Source: CAD feature listing. Evaluate the final solid. Frame: model axes, mm. Face numbers are marked on the shaded views. A direction names the side the tool comes from. Round coordinates to 2 decimals unless told otherwise and drop trailing zeros. Order: outer loops, then holes, each group sorted by start corner. A loop starts at its lowest first (then second) coordinate and runs counter-clockwise, first axis right, second up. Notation, with made-up numbers: M 80,22 L 125,22 A20 cw 125,51 Z; hole C 65.5,15 d2. An arc over 180 degrees is marked long. Answer as CSV lines item,"result". Start each with the question number.
Item 1: Section query C-C on y = 15. Return the cut outline in (x, z), plus the area to 3 significant figures.
Item 2: Set-up query: the marked faces 1 and 2. Return all of +Z, -Z, +X, -X, +Y, -Y with unobstructed straight access to the full face (end or side cutting, diameter ignored); none if empty.
Item 3: Pull-direction query (Z, two-part tool) for the marked faces 3, 4, 5 and 6; classes: +Z half, -Z half, draft (parallel to the pull), parting line (faces both ways), or undercut.
Item 4: Section query A-A on z = 43. Return the cut outline in (x, y), plus the area to 3 significant figures.
Item 5: Line query: line 1 (Y direction, x = -12.5, z = 23); line 2 (Y direction, x = -20, z = 2). Output: solid intervals per line, ascending. Write a range as [from, to].
Item 6: Section query B-B on x = 0. Return the cut outline in (y, z), plus the area to 3 significant figures.
Item 7: First-contact query: P1, Ø2.5, axis at y = 11.5, z = 2.5, coming from the +X side; P2, Ø1.1, axis at x = 27, z = 16, coming from the +Y side; P3, Ø3, axis at x = 20, y = 15, coming from the +Z side; P4, Ø4, axis at x = 9.9, z = 52.9, coming from the +Y side. Flat tips, straight axial feed; report the tip coordinate or a pass-through.
Item 8: Section query D-D on y = 23.25. Return the cut outline in (x, z).
from build123d import *

# Parameters (mm, degrees)
SKETCH016_W         = 54
SKETCH016_H         = 20
SKETCH016_R         = 2.35
PAD010_DEPTH        = 5
SKETCH019_R         = 11.1
SKETCH019_R_2       = 1.65
PAD009_DEPTH        = 10
SKETCH017_R         = 32.6
POCKET006_DEPTH     = 15.001
SKETCH076_R         = 32.6
SKETCH076_R_2       = 28.75
PAD049_DEPTH        = 4
SKETCH090_R         = 1.092
PAD055_DEPTH        = 26.5
HOLE009_D           = 3.4
HOLE009_CSINK_D     = 6.7
HOLE009_CSINK_ANGLE = 90


with BuildPart() as part:
    # Sketch016 → Pad010 (new body)
    with BuildSketch(Plane.XY):
        with Locations((0, 10)):
            Rectangle(SKETCH016_W, SKETCH016_H)
        with Locations((-20, 15)):
            Circle(SKETCH016_R, mode=Mode.SUBTRACT)
        with Locations((20, 15)):
            Circle(SKETCH016_R, mode=Mode.SUBTRACT)
    extrude(amount=PAD010_DEPTH)

    # Sketch019 → Pad009 (join)
    with BuildSketch(Plane.XZ):
        with BuildLine():
            Line((-27, 5), (-34.41436, 34.287835))
            ThreePointArc((34.41436, 34.287835), (0, 78.5), (-34.41436, 34.287835))
            Line((34.41436, 34.287835), (27, 5))
            Line((-27, 5), (27, 5))
        make_face()
        with Locations((0, 43)):
            Circle(SKETCH019_R, mode=Mode.SUBTRACT)
        with Locations((9.899495, 52.899495)):
            Circle(SKETCH019_R_2, mode=Mode.SUBTRACT)
        with Locations((-9.899495, 52.899495)):
            Circle(SKETCH019_R_2, mode=Mode.SUBTRACT)
        with Locations((9.899495, 33.100505)):
            Circle(SKETCH019_R_2, mode=Mode.SUBTRACT)
        with Locations((-9.899495, 33.100505)):
            Circle(SKETCH019_R_2, mode=Mode.SUBTRACT)
    extrude(amount=-PAD009_DEPTH)

    # Sketch017 → Pocket006 (cut, through all)
    with BuildSketch(Plane.XZ.offset(-5)):
        with Locations((0, 43)):
            Circle(SKETCH017_R)
    extrude(amount=-POCKET006_DEPTH, mode=Mode.SUBTRACT)

    # Sketch076 → Pad049 (join)
    with BuildSketch(Plane.XZ.offset(-4)):
        with Locations((0, 43)):
            Circle(SKETCH076_R)
        with Locations((0, 43)):
            Circle(SKETCH076_R_2, mode=Mode.SUBTRACT)
    extrude(amount=-PAD049_DEPTH)

    # Sketch090 → Pad055 (join)
    with BuildSketch(Plane.XZ):
        Polygon((28.284271, 24.615224), (23.334524, 19.665476), (23.334524, 12.594408), (32.526912, 3.40202), (41.012193, 11.887302), align=None)
        with Locations((32.526912, 10.473088)):
            Circle(SKETCH090_R, mode=Mode.SUBTRACT)
        with Locations((26.870058, 16.129942)):
            Circle(SKETCH090_R, mode=Mode.SUBTRACT)
    extrude(amount=-PAD055_DEPTH)

    # Hole009 (through all)
    with Locations(Plane(origin=(0, 5, 0), x_dir=(1, 0, 0), z_dir=(0, 1, 0))):
        with Locations((-9.899495, -52.899495), (9.899495, -52.899495), (9.899495, -33.100505), (-9.899495, -33.100505)):
            CounterSinkHole(HOLE009_D / 2, HOLE009_CSINK_D / 2, counter_sink_angle=HOLE009_CSINK_ANGLE)


solid = part.part
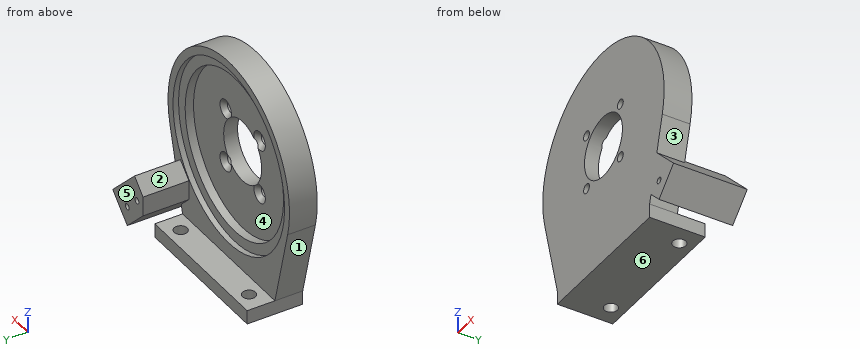
Results:
1,outline,"M -27,0 L -22.35,0 L -22.35,5 L -27,5 Z; M -17.65,0 L 17.65,0 L 17.65,5 L -17.65,5 Z; M 22.35,0 L 27,0 L 27,5 L 22.35,5 Z; M 23.33,12.59 L 32.53,3.4 L 41.01,11.89 L 28.28,24.62 L 23.33,19.67 Z; hole C 26.87,16.13 d2.18; hole C 32.53,10.47 d2.18"
1,area,"419 mm^2"
2,face 1,"-Z, -X, +Y, -Y"
2,face 2,"+Z, -X, +Y"
3,face 3,"undercut"
3,face 4,"undercut"
3,face 5,"draft"
3,face 6,"-Z half"
4,outline,"M -35.5,0 L -11.1,0 L -11.1,5 L -28.75,5 L -28.75,8 L -32.6,8 L -32.6,10 L -35.5,10 Z; M 11.1,0 L 35.5,0 L 35.5,10 L 32.6,10 L 32.6,8 L 28.75,8 L 28.75,5 L 11.1,5 Z"
4,area,"296 mm^2"
5,line 1,"[0, 5]"
5,line 2,"[0, 12.65], [17.35, 20]"
6,outline,"M 0,0 L 20,0 L 20,5 L 10,5 L 10,10.4 L 8,10.4 L 8,14.25 L 5,14.25 L 5,31.9 L 0,31.9 Z; M 0,54.1 L 5,54.1 L 5,71.75 L 8,71.75 L 8,75.6 L 10,75.6 L 10,78.5 L 0,78.5 Z"
6,area,"421 mm^2"
7,P1,"x = 32.87"
7,P2,"y = 10"
7,P3,"through"
7,P4,"y = 3.65"
8,outline,"M 23.33,12.59 L 32.53,3.4 L 41.01,11.89 L 28.28,24.62 L 23.33,19.67 Z; hole C 26.87,16.13 d2.18; hole C 32.53,10.47 d2.18"
